Model file for the job. Use its own axes, mm. Face numbers are marked on the shaded views. Round coordinates to 2 decimals unless told otherwise and drop trailing zeros. Order: outer loops, then holes, each group sorted by start corner. A loop starts at its lowest first (then second) coordinate and runs counter-clockwise, first axis right, second up. Notation, with made-up numbers: (-20.75, 39.25) - (10.25, 39.25) arc R22 cw to (10.25, 67.25) - close; hole circle Ø5 at (80.25, 85). An arc over 180 degrees is marked (long way). Use one line per item in the form item = value.
Autodesk Inventor part; units mm, degrees
ref_plane "XZ Plane" through (0, 0, 0) normal (0, 1, 0) x (-1, 0, 0)
ref_plane "XY Plane" through (0, 0, 0) normal (0, 0, 1) x (1, 0, 0)
sketch "Skizze1" plane through (0, 0, 0) normal (0, 0, 1) x (1, 0, 0)
  circle A0 centre (0, 0) radius 31
  circle A1 centre (0, 0) radius 30
  dimension "d0" = 62
  dimension "d1" = 60
extrude "Extrusion1" add sketch "Skizze1" along normal mid plane 300
ref_plane "Arbeitsebene1" through (30.5, 0, 0) normal (1, 0, 0) x (0, 1, 0)
sketch "Skizze2" plane through (30.5, 0, 0) normal (1, 0, 0) x (0, 1, 0)
  circle A0 centre (0, 144) radius 1.75
  line L0 (31, 150) -> (-31, 150)
  point P0 (0, 0)
  dimension "d5" = 3.5
  dimension "d6" = 6
extrude "Extrusion2" cut sketch "Skizze2" against normal mid plane 10
mirror "Spiegeln1" about plane through (0, 0, 0) normal (0, 0, 1) of "Extrusion2"
properties part number "Segment_elektro"
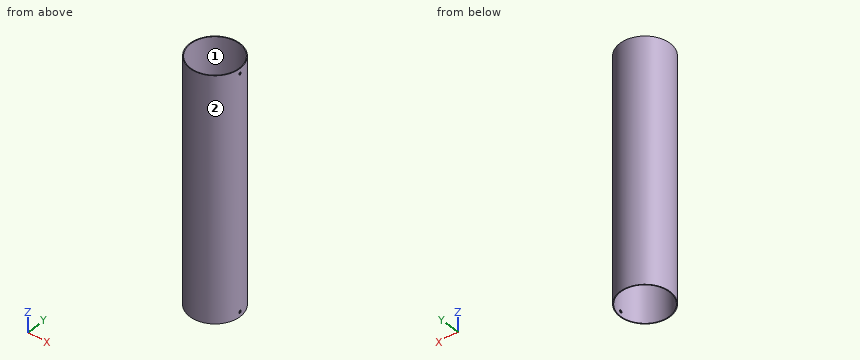
(1) Slice it at B-B on y = -5.5. Give the cut face in (x, z).
Report:
outline = (-30.51, -150) - (-29.49, -150) - (-29.49, 150) - (-30.51, 150) - close; (29.49, -150) - (30.51, -150) - (30.51, 150) - (29.49, 150) - close
(2) Pin check, flat tips, straight feed: pin 1 (1 mm diameter, centred on x = -8, z = 89, fed in from -Y); pin 2 (12 mm diameter, centred on x = -14.5, z = -105, fed in from -Y); pin 3 (12 mm diameter, centred on y = 19, z = 92, fed in from +X). Stop position of each tip, or through.
Report:
pin_1 = -30.08
pin_2 = -29.81
pin_3 = 28.14
(3) Slice it at C-C on z = -114. Give the cut face in (x, y), then the cut area to 3 significant figures.
Report:
outline = circle Ø62 at (0, 0); hole circle Ø60 at (0, 0)
area = 192 mm2
(4) Probe probe 1 along Z at (x, y) = (30.3, 0); probe 2 along Y at (x, z) = (0, 17); probe 3 along X at (y, z) = (-26.5, -112). List the from-to ranges inside material, lowest first. Write a range as [from, to].
Report:
probe_1 = [-150, -145.75], [-142.25, 142.25], [145.75, 150]
probe_2 = [-31, -30], [30, 31]
probe_3 = [-16.09, -14.06], [14.06, 16.09]
(5) Slice it at A-A on x = 0. Give the cut face in (y, z), then the cut area to 3 significant figures.
Report:
outline = (-31, -150) - (-30, -150) - (-30, 150) - (-31, 150) - close; (30, -150) - (31, -150) - (31, 150) - (30, 150) - close
area = 600 mm2
(6) Pull direction X, two halves, no side cores. Call the marked faces 1 and 2: released by +X, released by -X, zero draft, split by the parting line, or undercut.
Report:
face_1 = undercut
face_2 = split by the parting line
